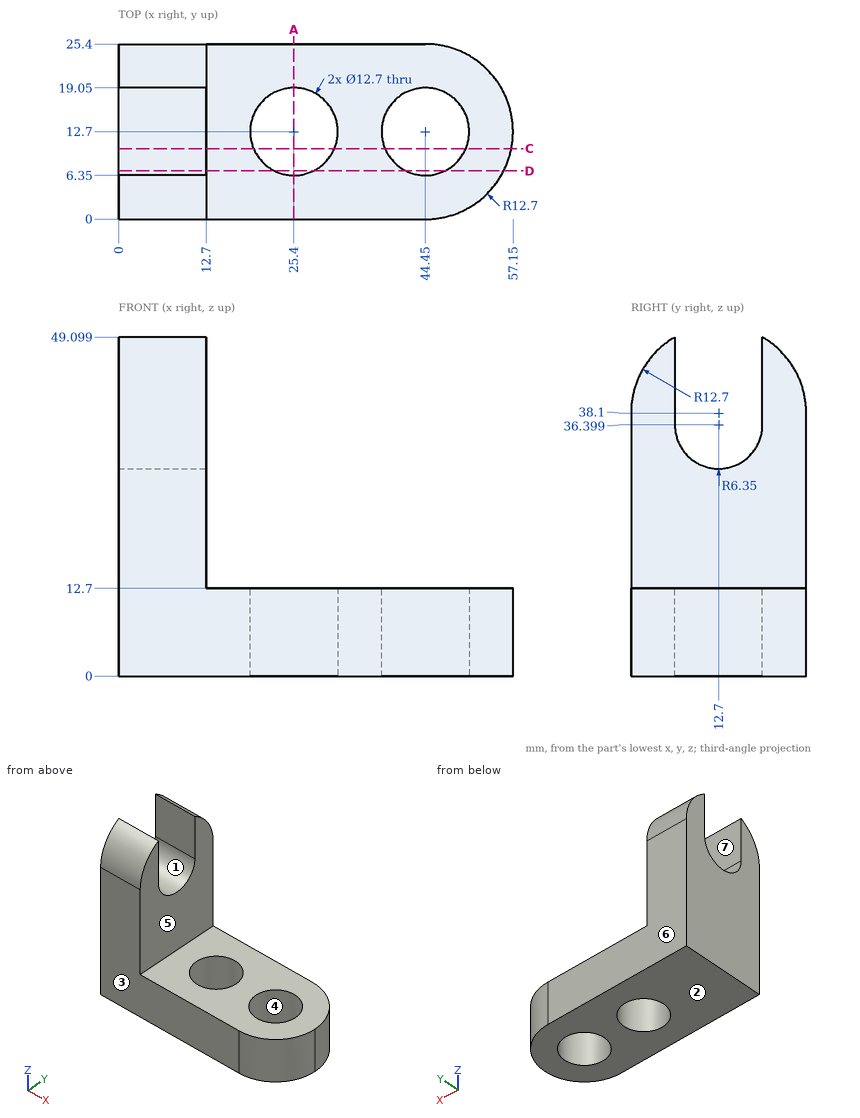
The figure shows three views and two pictorial views of one solid part (mm, origin at its lowest corner). Answer the questions. A direction names the side the tool comes from. Give positions to 0.01 mm unless a question says otherwise; leave off trailing zeros. Write each loop counter-clockwise with the first axis right and the second up, starting at its lowest first coordinate (ties: lowest second). Pieces come first, ordered by that corner, then holes. Notation, with made-up numbers: (-3.5, 44) - (7.5, 44) arc R18 ccw to (7.5, 68) - close; hole circle Ø7 at (-20, 53.25). An arc over 180 degrees is marked (long way). Return JSON: item names as keys, results as strings.
Q1. For a pull along Y with two mould halves and no side action, classify the marked faces 1, 2, 3 and 4 as released by +Y, released by -Y, zero draft, split by the parting line, or undercut.
Reply:
{"face 1": "undercut", "face 2": "zero draft", "face 3": "released by -Y", "face 4": "undercut"}
Q2. A cutting plane is placed at D-D, the plane y = 7. Determine the outline of the cut face in (x, z), and give its area (3 significant figures).
Reply:
{"outline": "(0, 0) - (22.6, 0) - (22.6, 12.7) - (12.7, 12.7) - (12.7, 33.6) - (0, 33.6) - close; (28.2, 0) - (41.65, 0) - (41.65, 12.7) - (28.2, 12.7) - close; (47.25, 0) - (55.8, 0) - (55.8, 12.7) - (47.25, 12.7) - close", "area": "832 mm²"}
Q3. A cutting plane is placed at C-C, the plane y = 10.25. Determine the outline of the cut face in (x, z).
Reply:
{"outline": "(0, 0) - (19.54, 0) - (19.54, 12.7) - (12.7, 12.7) - (12.7, 30.54) - (0, 30.54) - close; (31.26, 0) - (38.59, 0) - (38.59, 12.7) - (31.26, 12.7) - close; (50.31, 0) - (56.91, 0) - (56.91, 12.7) - (50.31, 12.7) - close"}
Q4. A cutting plane is placed at A-A, the plane x = 25.4. Determine the outline of the cut face in (y, z).
Reply:
{"outline": "(0, 0) - (6.35, 0) - (6.35, 12.7) - (0, 12.7) - close; (19.05, 0) - (25.4, 0) - (25.4, 12.7) - (19.05, 12.7) - close"}
Q5. For the marked faces 5, 6 and 7, determine the directions among +Z, -Z, +X, -X, +Y, -Y from which every point of the face is accessible in a straight line to the end or side of a thin tool.
Reply:
{"face 5": "+Z, +X, +Y, -Y", "face 6": "+Z, -Z, +X, -X, +Y", "face 7": "+Z, +X, -X"}
Q6. Given P1, Ø1.5, axis at x = 17, y = 17, coming from the +Z side; P2, Ø12.5, axis at y = 8, z = 23, coming from the +X side; P3, Ø10, axis at x = 6, z = 45.5, coming from the -Y side, each flat-ended and moving along its own axis, determine where each tip first touches the part or whether it passes through.
Reply:
{"P1": "z = 12.7", "P2": "x = 12.7", "P3": "y = 0.23"}
Q7. Consider line 1 along Y through (x, z) = (25, 6); line 2 along X through (y, z) = (24.25, 34.5). Determine where each line is inside the solid, lowest interval first. Write a range as [from, to].
Reply:
{"line 1": "[0, 6.36], [19.04, 25.4]", "line 2": "[0, 12.7]"}
